Source: CAD feature listing. Evaluate the final solid. Frame: model axes, mm. A direction names the side the tool comes from. Coordinates: 2 decimals unless noted, no trailing zeros. Write each loop counter-clockwise with the first axis right and the second up, starting at its lowest first coordinate (ties: lowest second). Pieces come first, ordered by that corner, then holes. Notation, with made-up numbers: (39.25, 49.25) - (43.25, 49.25) arc R18 ccw to (43.25, 59.25) - close; hole circle Ø6 at (73, -35.75). An arc over 180 degrees is marked (long way). One line per question, with ' | ' between items.
from build123d import *

# Parameters (mm, degrees)
SKETCH1_W           = 80
SKETCH1_H           = 115
BOSS_EXTRUDE1_DEPTH = 20
SKETCH2_W           = 60
SKETCH2_H           = 15
BOSS_EXTRUDE2_DEPTH = 20
SKETCH4_W           = 10
SKETCH4_H           = 10
SKETCH4_W_2         = 5
SKETCH4_H_2         = 15
BOSS_EXTRUDE3_DEPTH = 10
SKETCH3_R           = 1.5
CUT_EXTRUDE1_DEPTH  = 15
SKETCH6_R           = 1.5
CUT_EXTRUDE3_DEPTH  = 15
SKETCH7_R           = 1.5
CUT_EXTRUDE4_DEPTH  = 136.157942631
SKETCH8_W           = 60
SKETCH8_H           = 95
CUT_EXTRUDE5_DEPTH  = 15
SKETCH9_W           = 7.6
SKETCH9_H           = 4.9
CUT_EXTRUDE6_DEPTH  = 158.970880442
SKETCH10_W          = 10.4
SKETCH10_H          = 7.8
CUT_EXTRUDE7_DEPTH  = 160.257246025
FILLET1_R           = 6
FILLET2_R           = 6
FILLET3_R           = 6
FILLET4_START       = -25
FILLET4_DEPTH       = 22


with BuildPart() as part:
    # Sketch1 → Boss-Extrude1 (new body)
    with BuildSketch(Plane.XY):
        with Locations((15.793103448, -40.120689655)):
            Rectangle(SKETCH1_W, SKETCH1_H)
    extrude(amount=BOSS_EXTRUDE1_DEPTH)

    # Sketch2 → Boss-Extrude2 (add)
    with BuildSketch(Plane.ZY.offset(24.206896552)):
        with Locations((50, -15.120689655)):
            Rectangle(SKETCH2_W, SKETCH2_H)
        Polygon((80, -7.620689655), (80, -22.620689655), (80, -62.620689655), (80, -77.620689655), (95, -77.620689655), (95, -7.620689655), align=None)
        with Locations((50, -70.120689655)):
            Rectangle(SKETCH2_W, SKETCH2_H)
    extrude(amount=-BOSS_EXTRUDE2_DEPTH)

    # Sketch4 → Boss-Extrude3 (add)
    with BuildSketch(Plane(origin=(-4.206896552, 0, 0), x_dir=(0, 0, -1), z_dir=(1, 0, 0))):
        with Locations((-90, -18.620689655)):
            Rectangle(SKETCH4_W, SKETCH4_H)
        with Locations((-92.5, -42.120689655)):
            Rectangle(SKETCH4_W_2, SKETCH4_H_2)
    extrude(amount=BOSS_EXTRUDE3_DEPTH)

    # Sketch3 → Cut-Extrude1 (cut)
    with BuildSketch(Plane.XY.offset(95)):
        with Locations((0.707744923, -18.620689655)):
            Circle(SKETCH3_R)
        with Locations((-20.292255077, -18.620689655)):
            Circle(SKETCH3_R)
        with Locations((-19.206896552, -29.620689655)):
            Circle(SKETCH3_R)
        with Locations((-19.206896552, -54.620689655)):
            Circle(SKETCH3_R)
        with Locations((-9.206896552, -42.120689655)):
            Circle(SKETCH3_R)
    extrude(amount=-CUT_EXTRUDE1_DEPTH, mode=Mode.SUBTRACT)

    # Sketch6 → Cut-Extrude3 (cut)
    with BuildSketch(Plane(origin=(0, -7.620689655, 0), x_dir=(1, 0, 0), z_dir=(0, 1, 0))):
        with Locations(Location((-19.206896552, -85, 0), (0, 0, 180))):
            Circle(SKETCH6_R)
        with Locations(Location((-19.206896552, -45, 0), (0, 0, 180))):
            Circle(SKETCH6_R)
    extrude(amount=-CUT_EXTRUDE3_DEPTH, mode=Mode.SUBTRACT)

    # Sketch7 → Cut-Extrude4 (cut, through all)
    with BuildSketch(Plane.XY.offset(20)):
        with Locations((10.793103448, -77.620689655)):
            Circle(SKETCH7_R)
        with Locations((10.793103448, -37.620689655)):
            Circle(SKETCH7_R)
        with Locations((10.793103448, -70.620689655)):
            Circle(SKETCH7_R)
        with Locations((10.793103448, -30.620689655)):
            Circle(SKETCH7_R)
        with Locations((10.793103448, -63.620689655)):
            Circle(SKETCH7_R)
        with Locations((10.793103448, -23.620689655)):
            Circle(SKETCH7_R)
    extrude(amount=-CUT_EXTRUDE4_DEPTH, mode=Mode.SUBTRACT)

    # Sketch8 → Cut-Extrude5 (cut)
    with BuildSketch(Plane.XY.offset(20)):
        with Locations((25.793103448, -50.120689655)):
            Rectangle(SKETCH8_W, SKETCH8_H)
    extrude(amount=-CUT_EXTRUDE5_DEPTH, mode=Mode.SUBTRACT)

    # Sketch9 → Cut-Extrude6 (cut, through all)
    with BuildSketch(Plane(origin=(55.793103448, 0, 0), x_dir=(0, 0, -1), z_dir=(1, 0, 0))):
        Polygon((-6.8, 12.479310345), (-14.4, 12.479310345), (-17.2, 12.479310345), (-17.2, 6.979310345), (-3.8, 6.979310345), (-3.8, 12.479310345), align=None)
        with Locations((-10.6, 14.929310345)):
            Rectangle(SKETCH9_W, SKETCH9_H)
    extrude(amount=-CUT_EXTRUDE6_DEPTH, mode=Mode.SUBTRACT)

    # Sketch10 → Cut-Extrude7 (cut, through all)
    with BuildSketch(Plane.XZ.offset(97.620689655)):
        with Locations((-19.006896552, 10.3)):
            Rectangle(SKETCH10_W, SKETCH10_H)
    extrude(amount=-CUT_EXTRUDE7_DEPTH, mode=Mode.SUBTRACT)

    # Fillet1
    fillet1_edges = [part.edges().sort_by_distance(p)[0] for p in [
        (-24.206896552, -77.620689655, 57.5),
    ]]
    fillet(fillet1_edges, radius=FILLET1_R)

    # Fillet2
    fillet2_edges = [part.edges().sort_by_distance(p)[0] for p in [
        (-4.206896552, -77.620689655, 57.5),
    ]]
    fillet(fillet2_edges, radius=FILLET2_R)

    # Fillet3
    fillet3_edges = [part.edges().sort_by_distance(p)[0] for p in [
        (-4.206896552, -7.620689655, 57.5),
    ]]
    fillet(fillet3_edges, radius=FILLET3_R)

    # Fillet4: read off the stored shape, not the designer's step
    # Fillet4 outline → Fillet4 (cut)
    with BuildSketch(Plane.YZ.offset(FILLET4_START)):
        with BuildLine():
            Line((-77.620689655, 95), (-77.620689655, 89))
            add(Edge.make_bspline(
                [(-77.620689655, 89), (-77.620689655, 95), (-71.620689655, 95)],
                knots=[0, 0, 0, 1, 1, 1], degree=2, weights=[1, 0.707106781, 1]))
            Line((-71.620689655, 95), (-77.620689655, 95))
        make_face()
    extrude(amount=FILLET4_DEPTH, mode=Mode.SUBTRACT)


solid = part.part
Item 1: Cut plane B-B on z = 45. Return loops of the section in (x, y).
Check sheet entries:
outline: (-24.21, -71.62) arc R6 ccw to (-18.21, -77.62) - (-10.21, -77.62) arc R6 ccw to (-4.21, -71.62) - (-4.21, -62.62) - (-24.21, -62.62) - close; (-24.21, -22.62) - (-20.71, -22.62) - (-20.71, -7.62) - (-24.21, -7.62) - close; (-17.71, -22.62) - (-4.21, -22.62) - (-4.21, -13.62) arc R6 ccw to (-10.21, -7.62) - (-17.71, -7.62) - close
Item 2: Mould query, pull axis Y, two halves, no side actions, for faces 1 (the face through (15, -39, 0)), 2 (the face through (1, -13.621, 90)), 3 (the face through (10.598, -29.133, 2.535)). Classes: pulls with the +Y half, pulls with the -Y half, needs draft (parallel to the pull), parting line crosses it, or undercut.
Check sheet entries:
face 1: needs draft | face 2: pulls with the +Y half | face 3: undercut
Item 3: Ray query, line 1 along Z through (x, y) = (-20.5, -49.5); line 2 along Z through (x, y) = (-18, -11); line 3 along Z through (x, y) = (24, -40). Return the intervals inside material, ascending. Write a range as [from, to].
Check sheet entries:
line 1: [0, 6.4], [14.2, 20], [80, 95] | line 2: [0, 6.4], [14.2, 44.11], [45.89, 84.11], [85.89, 95] | line 3: [0, 5]
Item 4: Access query for faces 4 (the face through (-17, -7.621, 58)), 5 (the face through (-14, -77.621, 54)), 6 (the face through (-19, -22.621, 85)), 7 (the face through (-21.79, -18.55, 87.6)), 8 (the face through (21, 15, 6.8)). Directions: +Z, -Z, +X, -X, +Y, -Y. A direction counts if a zero-diameter tool reaches every point of the face in a straight line with its end or side. Return the directions, or none.
Check sheet entries:
face 4: +Z, +X, -X, +Y | face 5: +Z, +X, -X, -Y | face 6: +Y | face 7: +Z | face 8: +X, -X, +Y
Item 5: Pin query (flat end, axial travel): pin 1 Ø1 at (x, y) = (34.5, -7) entering from -Z; pin 2 Ø12 at (x, z) = (-0.5, 66.5) entering from +Y; pin 3 Ø1.8 at (x, y) = (10.79, -23.62) entering from -Z; pin 4 Ø12 at (x, z) = (39.5, 16) entering from -Y. Return the tip coordinate at first contact, or that it passes through.
Check sheet entries:
pin 1: z = 0 | pin 2: y = -8.9 | pin 3: through | pin 4: y = -2.62
Item 6: Cut plane C-C on x = 33. Return loops of the section in (y, z).
Check sheet entries:
outline: (-97.62, 0) - (17.38, 0) - (17.38, 6.8) - (12.48, 6.8) - (12.48, 3.8) - (6.98, 3.8) - (6.98, 17.2) - (12.48, 17.2) - (12.48, 14.4) - (17.38, 14.4) - (17.38, 20) - (-2.62, 20) - (-2.62, 5) - (-97.62, 5) - close
Item 7: Cut plane A-A on z = 71.5. Return loops of the section in (x, y).
Check sheet entries:
outline: (-24.21, -71.62) arc R6 ccw to (-18.21, -77.62) - (-10.21, -77.62) arc R6 ccw to (-4.21, -71.62) - (-4.21, -62.62) - (-24.21, -62.62) - close; (-24.21, -22.62) - (-4.21, -22.62) - (-4.21, -13.62) arc R6 ccw to (-10.21, -7.62) - (-24.21, -7.62) - close
